Read the model definition and answer for the solid it produces. Units are mm, in the model's axes. Give positions to 0.01 mm unless a question says otherwise; leave off trailing zeros. Loops run counter-clockwise (first coordinate to the right, second up) from the corner with the lowest first, then second, coordinate; pieces in that order, holes last. Notation, with made-up numbers: (74.5, -34) - (131.5, -34) arc R22 cw to (131.5, -3) - close; hole circle Ø2 at (53, 61.5). An arc over 180 degrees is marked (long way). Write item = value, one per line.
```python
from build123d import *

# Parameters (mm, degrees)
F0_W     = 90
F0_H     = 3.3
F1_DEPTH = 2.4
F2_T     = -1.2
F3_R     = 0.3


with BuildPart() as f1:
    # F0 (on Front) → F1 (new body)
    with BuildSketch(Plane.XZ):
        with Locations((45, 1.65)):
            Rectangle(F0_W, F0_H)
    extrude(amount=F1_DEPTH)

    # F2
    f2_openings = [f1.faces().sort_by_distance(p)[0] for p in [
        (45, -2.4, 1.65),
        (90, -1.2, 1.65),
        (0, -1.2, 1.65),
    ]]
    offset(amount=F2_T, openings=f2_openings)

    # F3
    f3_edges = [f1.edges().sort_by_distance(p)[0] for p in [
        (45, -2.4, 3.3),
        (45, 0, 3.3),
        (45, -2.4, 0),
        (45, 0, 0),
    ]]
    fillet(f3_edges, radius=F3_R)


solid = f1.part
```
1) Find the intervals of material crossed by probe 1 along Z at (x, y) = (23, -2); probe 2 along Z at (x, y) = (26.5, -2.3); probe 3 along Y at (x, z) = (6.5, 1.4), in increasing order.
Output:
probe_1 = 0 to 1.2, 2.1 to 3.3
probe_2 = 0.08 to 1.2, 2.1 to 3.22
probe_3 = -1.2 to 0
2) A cutting plane is placed at B-B on x = 8. Determine the outline of the cut face in (y, z), then the cut area to 3 significant figures.
Output:
outline = (-2.4, 0.3) arc R0.3 ccw to (-2.1, 0) - (-0.3, 0) arc R0.3 ccw to (0, 0.3) - (0, 3) arc R0.3 ccw to (-0.3, 3.3) - (-2.1, 3.3) arc R0.3 ccw to (-2.4, 3) - (-2.4, 2.1) - (-1.2, 2.1) - (-1.2, 1.2) - (-2.4, 1.2) - close
area = 6.76 mm²
3) A cutting plane is placed at A-A on y = -1.6. Determine the outline of the cut face in (x, z), then the cut area to 3 significant figures.
Output:
outline = (0, 0) - (90, 0) - (90, 1.2) - (0, 1.2) - close; (0, 2.1) - (90, 2.1) - (90, 3.3) - (0, 3.3) - close
area = 216 mm²
